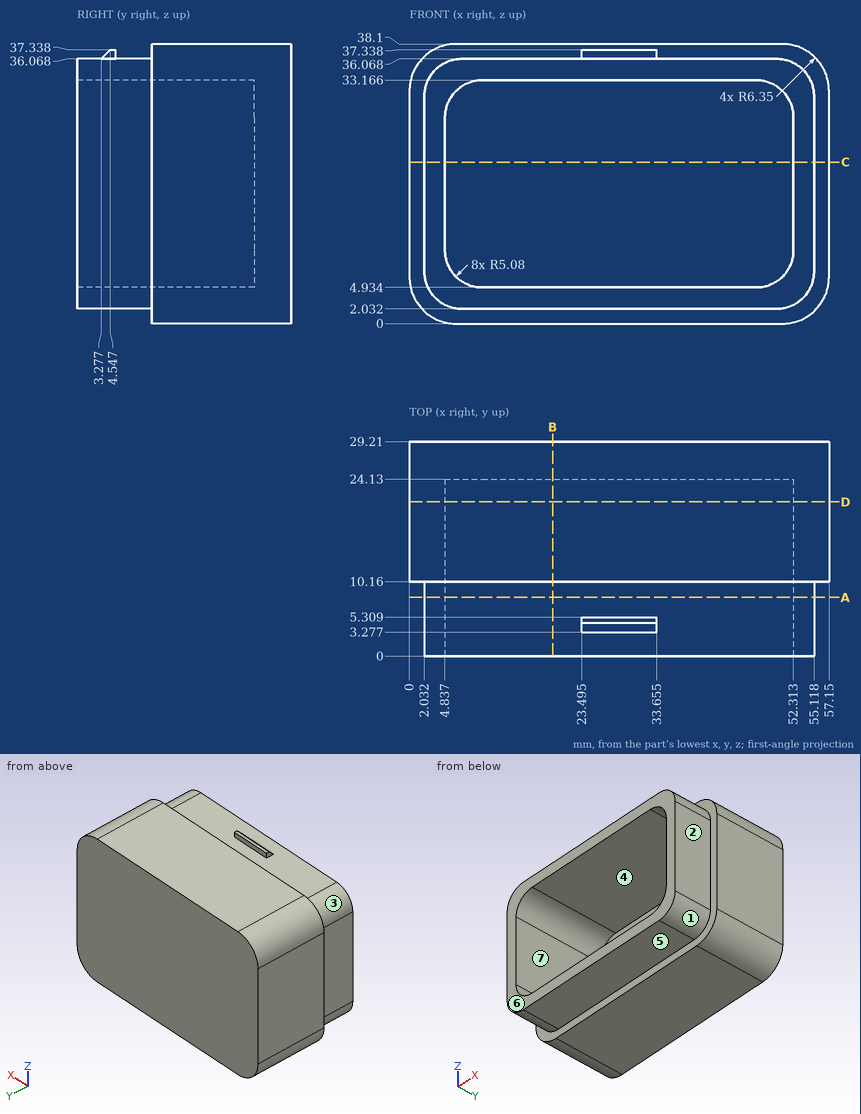
Answer from the drawing. Dimensions are ordinates in mm from the lowest x, y and z of the part. A direction names the side the tool comes from. Give positions to 0.01 mm unless a question says otherwise; leave off trailing zeros. Order: outer loops, then holes, each group sorted by start corner. A loop starts at its lowest first (then second) coordinate and runs counter-clockwise, first axis right, second up. Notation, with made-up numbers: (-13.5, -31.5) -> (44.5, -31.5) arc R15 ccw to (44.5, -6.5) -> close; hole circle Ø11 at (31, 28.25). An arc over 180 degrees is marked (long way). One line per item, written item: value. Start each with the question number.
(1) Straight lines are drawn through the part: L1, parallel to Z at x = 13, y = 13.5; L2, parallel to Z at x = 45, y = 2.5; L3, parallel to X at y = 19.5, z = 12. For each, find the intervals that lie inside material, in ascending order.
(2) For a pull along Z with two mould halves and no side action, classify the marked faces 5, 6 and 7 as released by +Z, released by -Z, zero draft, split by the parting line, or undercut.
(3) The part is cut by section C-C (z = 22). Determine the outline of the cut face in (x, y).
(4) The part is cut by section A-A (y = 8). Determine the outline of the cut face in (x, z).
(5) The part is cut by section D-D (y = 21). Determine the outline of the cut face in (x, z).
(6) A tool of negligible diameter and unlimited length cuts with its end or side. For the marked faces 1, 2, 3 and 4, from which of +Z, -Z, +X, -X, +Y, -Y can it reach the whole face along a straight path? Write none if from no direction.
(7) Flat-ended cylindrical pins translate along their axes: P1, Ø14, axis at x = 30, z = 25, coming from the -Y side; P2, Ø3, axis at y = 6.5, z = 14.5, coming from the +X side; P3, Ø0.6, axis at x = 31, y = 5, coming from the +Z side. Find the tip coordinate at first contact, or state that the pin passes through.
(8) The part is cut by section B-B (x = 19.5). Determine the outline of the cut face in (y, z).
Taken from the geometry:
1. L1: 0 to 4.93, 33.17 to 38.1
1. L2: 2.03 to 4.93, 33.17 to 36.07
1. L3: 0 to 4.84, 52.31 to 57.15
2. face 5: released by -Z
2. face 6: zero draft
2. face 7: undercut
3. outline: (0, 10.16) -> (2.03, 10.16) -> (2.03, 0) -> (4.84, 0) -> (4.84, 24.13) -> (52.31, 24.13) -> (52.31, 0) -> (55.12, 0) -> (55.12, 10.16) -> (57.15, 10.16) -> (57.15, 29.21) -> (0, 29.21) -> close
4. outline: (2.03, 7.11) arc R5.08 ccw to (7.11, 2.03) -> (50.04, 2.03) arc R5.08 ccw to (55.12, 7.11) -> (55.12, 30.99) arc R5.08 ccw to (50.04, 36.07) -> (7.11, 36.07) arc R5.08 ccw to (2.03, 30.99) -> close; hole (4.84, 10.01) arc R5.08 ccw to (9.92, 4.93) -> (47.23, 4.93) arc R5.08 ccw to (52.31, 10.01) -> (52.31, 28.09) arc R5.08 ccw to (47.23, 33.17) -> (9.92, 33.17) arc R5.08 ccw to (4.84, 28.09) -> close
5. outline: (0, 6.35) arc R6.35 ccw to (6.35, 0) -> (50.8, 0) arc R6.35 ccw to (57.15, 6.35) -> (57.15, 31.75) arc R6.35 ccw to (50.8, 38.1) -> (6.35, 38.1) arc R6.35 ccw to (0, 31.75) -> close; hole (4.84, 10.01) arc R5.08 ccw to (9.92, 4.93) -> (47.23, 4.93) arc R5.08 ccw to (52.31, 10.01) -> (52.31, 28.09) arc R5.08 ccw to (47.23, 33.17) -> (9.92, 33.17) arc R5.08 ccw to (4.84, 28.09) -> close
6. face 1: -Z, +X, -Y
6. face 2: +Z, -Z, +X, -Y
6. face 3: +Z, -X, -Y
6. face 4: -Y
7. P1: y = 24.13
7. P2: x = 55.12
7. P3: z = 37.34
8. outline: (0, 2.03) -> (10.16, 2.03) -> (10.16, 0) -> (29.21, 0) -> (29.21, 38.1) -> (10.16, 38.1) -> (10.16, 36.07) -> (0, 36.07) -> (0, 33.17) -> (24.13, 33.17) -> (24.13, 4.93) -> (0, 4.93) -> close
